```python
from build123d import *

# Parameters (mm, degrees)
F0_R      = 101.6
F0_R_2    = 44.45
F1_DEPTH  = 52.3875
F2_R      = 69.088
F3_DEPTH  = 92.075
F4_R      = 74.93
F5_DEPTH  = 69.85
F6_R      = 6.35
F7_R      = 1.5875
F9_D      = 10.71626
F9_DEPTH  = 25.3941384615
F9_TIP    = 3.2194893086
F10_W     = 294.4396436214
F10_H     = 108.7958868504
F11_DEPTH = 104.776
F12_W     = 161.925
F12_H     = 25.4
F13_DEPTH = 104.7760001
F15_D     = 14.2875
F17_R     = 12.7
F18_DEPTH = 88.1072501


with BuildPart() as f1:
    # F0 (on Right) → F1 (new body, symmetric)
    with BuildSketch(Plane.YZ):
        Circle(F0_R)
        Circle(F0_R_2, mode=Mode.SUBTRACT)
    extrude(amount=F1_DEPTH, both=True)

    # F2 (on face) → F3 (cut)
    with BuildSketch(Plane.YZ.offset(52.3875)):
        Circle(F2_R)
    extrude(amount=-F3_DEPTH, mode=Mode.SUBTRACT)

    # F4 (on face) → F5 (cut)
    with BuildSketch(Plane.YZ.offset(52.3875)):
        Circle(F4_R)
    extrude(amount=-F5_DEPTH, mode=Mode.SUBTRACT)

    # F6
    f6_edges = [f1.edges().sort_by_distance(p)[0] for p in [
        (-39.6875, -69.088, 0),
    ]]
    fillet(f6_edges, radius=F6_R)

    # F7
    f7_edges = [f1.edges().sort_by_distance(p)[0] for p in [
        (-17.4625, -74.93, 0),
    ]]
    fillet(f7_edges, radius=F7_R)

    # F9
    with Locations(Plane.YZ.offset(52.3875)):
        with Locations((-76.9896583964, 44.45), (0, 88.9), (76.9896583964, 44.45)):
            Hole(F9_D / 2, depth=F9_DEPTH)
            with Locations((0, 0, -(F9_DEPTH + F9_TIP / 2))):  # 118° drill point
                Cone(0, F9_D / 2, F9_TIP, mode=Mode.SUBTRACT)

    # F10 (on face) → F11 (cut, through all)
    with BuildSketch(Plane.YZ.offset(52.3875)):
        with Locations((-3.7660896778, -59.9541934252)):
            Rectangle(F10_W, F10_H)
    extrude(amount=-F11_DEPTH, mode=Mode.SUBTRACT)

    # F12 (on face) → F13 (cut, through all)
    with BuildSketch(Plane.YZ.offset(52.3875)):
        with Locations((0, -12.7)):
            Rectangle(F12_W, F12_H)
    extrude(amount=-F13_DEPTH, mode=Mode.SUBTRACT)

    # F15 (through all)
    with Locations(Plane(origin=(0, 0, -5.55625), x_dir=(1, 0, 0), z_dir=(0, 0, -1))):
        with Locations((15.8115, 90.4875), (-34.9885, 90.4875), (15.8115, -90.4875), (-34.9885, -90.4875)):
            Hole(F15_D / 2)

    # F17 (on offset) → F18 (cut, through all)
    with BuildSketch(Plane(origin=(0, 0, 13.49375), x_dir=(1, 0, 0), z_dir=(0, 0, -1))):
        with Locations((-34.9885, 90.4875)):
            Circle(F17_R)
        with Locations((15.8115, 90.4875)):
            Circle(F17_R)
        with Locations((-34.9885, -90.4875)):
            Circle(F17_R)
        with Locations((15.8115, -90.4875)):
            Circle(F17_R)
    extrude(amount=-F18_DEPTH, mode=Mode.SUBTRACT)


solid = f1.part
```
Verification items for the finished model (mm, model axes). A direction names the side the tool comes from. Round coordinates to 2 decimals unless told otherwise and drop trailing zeros. Write each loop counter-clockwise with the first axis right and the second up, starting at its lowest first coordinate (ties: lowest second). Pieces come first, ordered by that corner, then holes. Notation, with made-up numbers: (-17.5, 87) -> (33.5, 87) arc R14 cw to (33.5, 108) -> close; hole circle Ø8 at (6.25, 84). An arc over 180 degrees is marked (long way). Write each question's results on one line, items separated by ' | '. Start each with the question number.
1. Draft check along X on faces 1 (the cylindrical face through (-41.802, -92.633, 4.102)), 2 (the flat face through (1, 91, -5.556)), 3 (the flat face through (52.388, -8, 76)), 4 (the flat face through (-41, -84, 13.494)). Enter one of: +X half, -X half, draft (parallel to the pull), parting line (faces both ways), or undercut.
2. Cross-section at C-C (y = 88). Enter the section's corners in (x, z).
3. Depth check by flat-ended pin: P1, Ø4, axis at x = 41, z = 20.5, coming from the -Y side; P2, Ø11.5, axis at x = 12, y = -86, coming from the +Z side; P3, Ø1.7, axis at x = -5.5, z = -2, coming from the +Y side; P4, Ø11.5, axis at x = 15.81, y = -90.49, coming from the -Z side. Enter the tip coordinate at first touch or a pass-through.
4. Cross-section at A-A (y = -87). Enter the section's corners in (x, z).
5. Set-up check for faces 5 (the flat face through (1, 80.962, -3)), 6 (the flat face through (-39.688, -1, 46)), 7 (the cylindrical face through (39.51, 80.94, 48.07)), 8 (the cylindrical face through (21.48, -86.14, 4.1)), 9 (the cylindrical face through (16.257, 77.795, 33.304)): record each of +Z, -Z, +X, -X, +Y, -Y from which the full face is reachable in a straight line by a thin tool's end or side.
6. Cross-section at B-B (z = 10). Count the separate pieces of the cut face and the enclosed holes in it, then the cut area to 3 significant figures.
7. Material ranges on probe 1 along Z at (x, y) = (44.5, 0); probe 2 along Y at (x, z) = (-21.5, 21); probe 3 along X at (y, z) = (-64, 29), recorded low to high. Write a range as from..to.
Solutions:
1) face 1: undercut | face 2: draft | face 3: +X half | face 4: undercut
2) outline: (-52.39, -5.56) -> (-41.69, -5.56) -> (-41.69, 13.49) -> (-47.44, 13.49) -> (-47.44, 50.78) -> (-52.39, 50.78) -> close; (-28.29, -5.56) -> (9.11, -5.56) -> (9.11, 13.49) -> (3.36, 13.49) -> (3.36, 50.78) -> (-22.53, 50.78) -> (-22.53, 13.49) -> (-28.29, 13.49) -> close; (22.51, -5.56) -> (52.39, -5.56) -> (52.39, 50.78) -> (28.27, 50.78) -> (28.27, 13.49) -> (22.51, 13.49) -> close
3) P1: stops at y = -99.9 | P2: stops at z = 13.49 | P3: stops at y = 101.59 | P4: passes through
4) outline: (-52.39, -5.56) -> (-41.22, -5.56) -> (-41.22, 13.49) -> (-47.2, 13.49) -> (-47.2, 52.47) -> (-52.39, 52.47) -> close; (-28.75, -5.56) -> (9.58, -5.56) -> (9.58, 13.49) -> (3.6, 13.49) -> (3.6, 52.47) -> (-22.78, 52.47) -> (-22.78, 13.49) -> (-28.75, 13.49) -> close; (22.05, -5.56) -> (52.39, -5.56) -> (52.39, 52.47) -> (28.02, 52.47) -> (28.02, 13.49) -> (22.05, 13.49) -> close
5) face 5: -Z, +X, -X | face 6: -Z, +X | face 7: +X | face 8: +Z, -Z | face 9: +Z
6) separate pieces: 2 | enclosed holes: 4 | area: 6,050 mm2
7) probe 1: z = 74.93..83.54, 94.26..101.6 | probe 2: y = -99.41..-65.82, 65.82..99.41 | probe 3: x = -52.39..-17.46
